```python
from build123d import *

# Parameters (mm, degrees)
F1_DEPTH = 15
F2_R     = 1.5
F3_DEPTH = 4.4278798556


# Not quite as in the source:
# - a feature names something its author has since deleted; it is built from what else it names


with BuildPart() as f1:
    # F0 (on Top) → F1 (new body)
    with BuildSketch(Plane.XY):
        with BuildLine():
            Line((1.7011785064, -11.877588293), (-1.7096480171, -11.877588293))
            ThreePointArc((-1.7096480171, -11.877588293), (-11.1202848878, -4.5099073176), (-9.5, 7.3314391493))
            ThreePointArc((-9.5, 7.3314391493), (-9.5385768198, 8.2900827327), (-10.4622412473, 8.0306030295))
            ThreePointArc((-10.4622412473, 8.0306030295), (-13.1913649606, -6.4201767786), (-2.3021989036, -16.3044681486))
            Line((-2.3021989036, -16.3044681486), (2.2770734892, -16.2874199147))
            ThreePointArc((2.2770734892, -16.2874199147), (12.7428435218, -6.1893456412), (10.5841437277, 8.1927078148))
            ThreePointArc((10.5841437277, 8.1927078148), (9.5441810303, 8.3863903947), (9.5, 7.3294687371))
            ThreePointArc((9.5, 7.3294687371), (11.1173000284, -4.5140615908), (1.7011785064, -11.877588293))
        make_face()
    extrude(amount=F1_DEPTH)

    # F2 (on face) → F3 (cut, through all)
    with BuildSketch(Plane(origin=(0, -11.877588293, 0), x_dir=(-1, 0, 0), z_dir=(0, 1, 0))):
        with Locations((0, 7.5)):
            Circle(F2_R)
    extrude(amount=-F3_DEPTH, mode=Mode.SUBTRACT)


solid = f1.part
```
Can you work these out from the model? Positions are in its coordinate system, mm. A direction names the side the tool comes from. Give positions to 0.01 mm unless a question says otherwise; leave off trailing zeros. Loops run counter-clockwise (first coordinate to the right, second up) from the corner with the lowest first, then second, coordinate; pieces in that order, holes last. Notation, with made-up numbers: M 89,0.5 L 141,0.5 A27 ccw 141,37.5 Z; hole C 20.25,9.25 d3. An arc over 180 degrees is marked long. Answer in a Markdown table with one row per item.
1. Suppose I cut it at B-B on y = -3.5. Write out the boundary of the cut face in (x, z), plus the area to 3 significant figures.
Taken from the geometry:
| item | result |
|---|---|
| outline | M -13.86,0 L -11.48,0 L -11.48,15 L -13.86,15 Z; M 11.48,0 L 13.4,0 L 13.4,15 L 11.48,15 Z |
| area | 64.5 mm² |
2. If I drill on line 1 along Z through (x, y) = (0, -14.9); line 2 along Y through (x, z) = (11, 6.5); line 3 along Y through (x, z) = (0, 3.75), over which ranges is the centre line in solid material (lowest first)?
Taken from the geometry:
| item | result |
|---|---|
| line 1 | z = 0 to 6, 9 to 15 |
| line 2 | y = -9.77 to -4.79, 4.79 to 7.59 |
| line 3 | y = -16.3 to -11.88 |
3. Thinking about a two-plate mould opening in X: for faces 1 (the flat face through (-1.3, -12.1, 0)), 2 (the cylindrical face through (-9.526, 8.281, 7.395)), 3 (the cylindrical face through (12.674, -6.389, 7.395)), which applies, released by +X, released by -X, zero draft, split by the parting line, or undercut?
Taken from the geometry:
| item | result |
|---|---|
| face 1 | zero draft |
| face 2 | undercut |
| face 3 | released by +X |
4. Suppose I cut it at A-A on x = 0. Write out the boundary of the cut face in (y, z), plus the area to 3 significant figures.
Taken from the geometry:
| item | result |
|---|---|
| outline | M -16.3,0 L -11.88,0 L -11.88,6 L -16.3,6 Z; M -16.3,9 L -11.88,9 L -11.88,15 L -16.3,15 Z |
| area | 53.0 mm² |
5. For pin 1 Ø3 at (x, z) = (4, 5.5) entering from -Y; pin 2 Ø5 at (x, z) = (-7, 11.5) entering from -Y; pin 3 Ø1.5 at (y, z) = (-9, 5) entering from -X; pin 4 Ø2.5 at (x, z) = (0, 7.5) entering from -Y, each with a flat end and sliding along its axis, tell me the tip position at first contact or that it passes through.
Taken from the geometry:
| item | result |
|---|---|
| pin 1 | stops at y = -16.22 |
| pin 2 | stops at y = -15.62 |
| pin 3 | stops at x = -12.44 |
| pin 4 | passes through |
6. Suppose I cut it at C-C on z = 7.5. Write out the boundary of the cut face in (x, y).
Taken from the geometry:
| item | result |
|---|---|
| outline | M -10.46,8.03 A15.06 ccw -2.3,-16.3 L -1.5,-16.3 L -1.5,-11.88 L -1.71,-11.88 A12 cw -9.5,7.33 A0.61 ccw long Z; M 1.5,-16.29 L 2.28,-16.29 A15.86 ccw 10.58,8.19 A0.7 ccw long 9.5,7.33 A12 cw 1.7,-11.88 L 1.5,-11.88 Z |
7. Which directions (+Z, -Z, +X, -X, +Y, -Y) give clear straight access to the entire face, cutting with the end or side of a thin tool? Please do faces 4 (the cylindrical face through (11.182, -4.351, 7.395)), 5 (the flat face through (0, -11.878, 5.7)), 6 (the cylindrical face through (0, -14, 6)).
Taken from the geometry:
| item | result |
|---|---|
| face 4 | +Z, -Z |
| face 5 | +Z, -Z, +Y |
| face 6 | +Y, -Y |
8. Suppose I cut it at D-D on z = 2.5. Write out the boundary of the cut face in (x, y), plus the area to 3 significant figures.
Taken from the geometry:
| item | result |
|---|---|
| outline | M -10.46,8.03 A15.06 ccw -2.3,-16.3 L 2.28,-16.29 A15.86 ccw 10.58,8.19 A0.7 ccw long 9.5,7.33 A12 cw 1.7,-11.88 L -1.71,-11.88 A12 cw -9.5,7.33 A0.61 ccw long Z |
| area | 160 mm² |
